```python
from build123d import *

# Parameters (mm, degrees)
ESQUISSE1_W      = 80
ESQUISSE1_H      = 100.00000000000001
EXTRUSION1_DEPTH = 6
ESQUISSE2_R      = 8
ESQUISSE2_R_2    = 7.999999999999998
ESQUISSE2_R_3    = 2.5000000000000018
ESQUISSE2_R_4    = 2.4999999999999956
ESQUISSE2_R_5    = 2.4999999999999982
ESQUISSE2_R_6    = 2.499999999999995
EXTRUSION3_DEPTH = 129.20296408429877
CHANFREIN1_SIZE  = 2.5


with BuildPart() as part:
    # Esquisse1 → Extrusion1 (new body)
    with BuildSketch(Plane(origin=(0, 0, 0), x_dir=(0, 0, -1), z_dir=(1, 0, 0))):
        with Locations((40, 50.00000000000001)):
            Rectangle(ESQUISSE1_W, ESQUISSE1_H)
    extrude(amount=EXTRUSION1_DEPTH)

    # Esquisse2 → Extrusion3 (cut, through all)
    with BuildSketch(Plane(origin=(6, 0, 0), x_dir=(0, 0, -1), z_dir=(1, 0, 0))):
        with Locations((40, 77.00000000000001)):
            Circle(ESQUISSE2_R)
        with Locations((40, 30)):
            Circle(ESQUISSE2_R_2)
        with Locations((5, 80)):
            Circle(ESQUISSE2_R_3)
        with Locations((75.00000000000001, 80)):
            Circle(ESQUISSE2_R_4)
        with Locations((5.000000000000136, 67)):
            Circle(ESQUISSE2_R_3)
        with Locations((75.00000000000016, 67)):
            Circle(ESQUISSE2_R_4)
        with Locations((20, 5.000000000000004)):
            Circle(ESQUISSE2_R_5)
        with Locations(Location((60.00000000000098, 5.000000000000004, 0), (0, 0, 180))):
            Circle(ESQUISSE2_R_6)
        with BuildLine():
            Line((17.499999999999996, 88.00000000000001), (23.568323274845017, 88.00000000000001))
            ThreePointArc((23.568323274845017, 88.00000000000001), (25.703928765288133, 86.79968811227509), (25.788820129595685, 84.35135135135135))
            ThreePointArc((25.788820129595685, 84.35135135135135), (24.477533819987812, 73.12017478610468), (30.918918918918916, 63.8267708439111))
            ThreePointArc((30.918918918918916, 63.8267708439111), (31.713289101913404, 62.930930175710394), (32, 61.7684537882722))
            Line((32, 61.7684537882722), (32, 45.231546211727824))
            ThreePointArc((32, 45.231546211727824), (31.713289101913414, 44.069069824289635), (30.918918918918926, 43.17322915608893))
            ThreePointArc((30.918918918918926, 43.17322915608893), (24.001358501680507, 29.79150489634176), (31.265293026281448, 16.594594594594593))
            ThreePointArc((31.265293026281448, 16.594594594594593), (32.297001527984975, 13.788131503185623), (29.900495061637923, 12))
            Line((29.900495061637923, 12), (17.500000000000007, 12))
            ThreePointArc((17.500000000000007, 12), (15.73223304703364, 12.732233047033631), (15.00000000000001, 14.499999999999998))
            Line((15.00000000000001, 14.499999999999998), (15.000000000000002, 85.5))
            ThreePointArc((15.000000000000002, 85.5), (15.732233047033617, 87.26776695296638), (17.499999999999996, 88.00000000000001))
        make_face()
        with BuildLine():
            Line((65, 85.5), (65.00000000000001, 14.5))
            ThreePointArc((65.00000000000001, 14.5), (64.26776695296637, 12.732233047033631), (62.5, 12))
            Line((62.5, 12), (50.09950493836208, 12))
            ThreePointArc((50.09950493836208, 12), (47.702998472015025, 13.78813150318562), (48.73470697371855, 16.594594594594593))
            ThreePointArc((48.73470697371855, 16.594594594594593), (55.99864149831949, 29.79150489634175), (49.08108108108109, 43.17322915608893))
            ThreePointArc((49.08108108108109, 43.17322915608893), (48.286710898086596, 44.06906982428963), (48, 45.23154621172782))
            Line((48, 45.23154621172782), (48, 61.7684537882722))
            ThreePointArc((48, 61.7684537882722), (48.286710898086596, 62.930930175710394), (49.08108108108109, 63.8267708439111))
            ThreePointArc((49.08108108108109, 63.8267708439111), (55.52246618001219, 73.1201747861047), (54.2111798704043, 84.35135135135137))
            ThreePointArc((54.2111798704043, 84.35135135135137), (54.29607123471186, 86.7996881122751), (56.43167672515498, 88.00000000000001))
            Line((56.43167672515498, 88.00000000000001), (62.5, 88.00000000000001))
            ThreePointArc((62.5, 88.00000000000001), (64.26776695296637, 87.26776695296637), (65, 85.5))
        make_face()
    extrude(amount=-EXTRUSION3_DEPTH, mode=Mode.SUBTRACT)

    # Chanfrein1
    chanfrein1_edges = [part.edges().sort_by_distance(p)[0] for p in [
        (6, 5.000000000000004, -17.5),
        (6, 5.0000000000000036, -62.50000000000097),
    ]]
    chamfer(chanfrein1_edges, length=CHANFREIN1_SIZE)


solid = part.part
```
The model under review builds one solid part; all positions refer to its coordinate system, in mm. A direction names the side the tool comes from. Coordinates: 2 decimals unless noted, no trailing zeros. Loops run counter-clockwise (first coordinate to the right, second up) from the corner with the lowest first, then second, coordinate; pieces in that order, holes last. Notation, with made-up numbers: (-20.5, 4.25) -> (-6.5, 4.25) arc R20 ccw to (-6.5, 17.25) -> close; hole circle Ø10 at (27.25, 51). An arc over 180 degrees is marked (long way). Answer as CSV lines item,"result".
Item 1: Machinability: for faces 4 (the conical face through (3.621, 6.595, -62.08)), 5 (the cylindrical face through (3, 30, -56)), which of the approach directions +Z, -Z, +X, -X, +Y, -Y give a long, thin tool a straight path to every point of the face, cutting with its end or side? Answer none if there is none.
Results below:
face 4,"+X"
face 5,"+X, -X"
Item 2: Take a section at B-B, the plane y = 67. State the section outline as (x, z) points, and give its area (3 significant figures).
Results below:
outline,"(0, -80) -> (6, -80) -> (6, -77.5) -> (0, -77.5) -> close; (0, -72.5) -> (6, -72.5) -> (6, -65) -> (0, -65) -> close; (0, -52.49) -> (6, -52.49) -> (6, -27.51) -> (0, -27.51) -> close; (0, -15) -> (6, -15) -> (6, -7.5) -> (0, -7.5) -> close; (0, -2.5) -> (6, -2.5) -> (6, 0) -> (0, 0) -> close"
area,"270 mm2"
Item 3: Take a section at D-D, the plane y = 30. State the section outline as (x, z) points.
Results below:
outline,"(0, -80) -> (6, -80) -> (6, -65) -> (0, -65) -> close; (0, -56) -> (6, -56) -> (6, -48) -> (0, -48) -> close; (0, -32) -> (6, -32) -> (6, -24) -> (0, -24) -> close; (0, -15) -> (6, -15) -> (6, 0) -> (0, 0) -> close"
Item 4: Insertion check: pin 1 (4.5 mm diameter, centred on y = 5, z = -60, fed in from +X). The pin has a flat end and moves straight along its axis. Give the tip position at first contact, or say it passes through.
Results below:
pin 1,"passes through"
Item 5: Draft analysis for pull direction Z (two halves, no side actions). For faces 1 (the flat face through (3, 49, 0)), 2 (the flat face through (6, 51, -39)), 3 (the cylindrical face through (3.042, 12.713, -15.752)), state which applies: +Z half, -Z half, draft (parallel to the pull), parting line (faces both ways), or undercut.
Results below:
face 1,"+Z half"
face 2,"draft"
face 3,"undercut"
Item 6: Take a section at A-A, the plane z = -40. State the section outline as (x, y) points, and give its area (3 significant figures).
Results below:
outline,"(0, 0) -> (6, 0) -> (6, 22) -> (0, 22) -> close; (0, 38) -> (6, 38) -> (6, 69) -> (0, 69) -> close; (0, 85) -> (6, 85) -> (6, 100) -> (0, 100) -> close"
area,"408 mm2"
Item 7: For L1, parallel to Z at x = 0.65, y = 57.5; L2, parallel to Y at x = 1.9, z = -75; L3, parallel to Y at x = 0.65, z = -39.5, list the stretches that pass through material, from the lowest coordinate up.
Results below:
L1,"z = -80 to -65, -48 to -32, -15 to 0"
L2,"y = 0 to 64.5, 69.5 to 77.5, 82.5 to 100"
L3,"y = 0 to 22.02, 37.98 to 69.02, 84.98 to 100"
Item 8: Take a section at C-C, the plane y = 5. State the section outline as (x, z) points.
Results below:
outline,"(0, -80) -> (6, -80) -> (6, -65) -> (3.5, -62.5) -> (0, -62.5) -> close; (0, -57.5) -> (3.5, -57.5) -> (6, -55) -> (6, -25) -> (3.5, -22.5) -> (0, -22.5) -> close; (0, -17.5) -> (3.5, -17.5) -> (6, -15) -> (6, 0) -> (0, 0) -> close"
